Study the drawing (mm; zero at the part's minimum x, y, z) and answer. Round coordinates to 2 decimals unless told otherwise and drop trailing zeros. Write each loop counter-clockwise with the first axis right and the second up, starting at its lowest first coordinate (ties: lowest second). Pieces come first, ordered by that corner, then holes. Notation, with made-up numbers: (23, 60) - (75, 60) arc R25 cw to (75, 92) - close; hole circle Ø4 at (47.25, 55.25). An arc over 180 degrees is marked (long way). Return JSON: item names as keys, results as strings. Group by question number.
(1) Each of these flat-tipped pins is pushed along its axis until it touches: pin 1 (4 mm diameter, centred on x = 30, y = 20, fed in from +Z); pin 2 (8 mm diameter, centred on x = 30, y = 50, fed in from +Z). Where does it stop, or does it pass through?
(2) Section B-B, the plane z = 0.4 is taken. Give the number of separate pieces and of enclosed holes in the cut face, then the cut area to 3 significant figures.
(3) Section C-C, the plane y = 27.5 is taken. Write down the section's boundary in (x, z), then the cut area to 3 significant figures.
(4) Section A-A, the plane y = 59 is taken. Write down the section's boundary in (x, z), then the cut area to 3 significant figures.
(5) Find the intervals of material crossed by line 1 along X through (y, z) = (34.5, 1.45); line 2 along X through (y, z) = (51, 0.25), in increasing order. Write a range as [from, to].
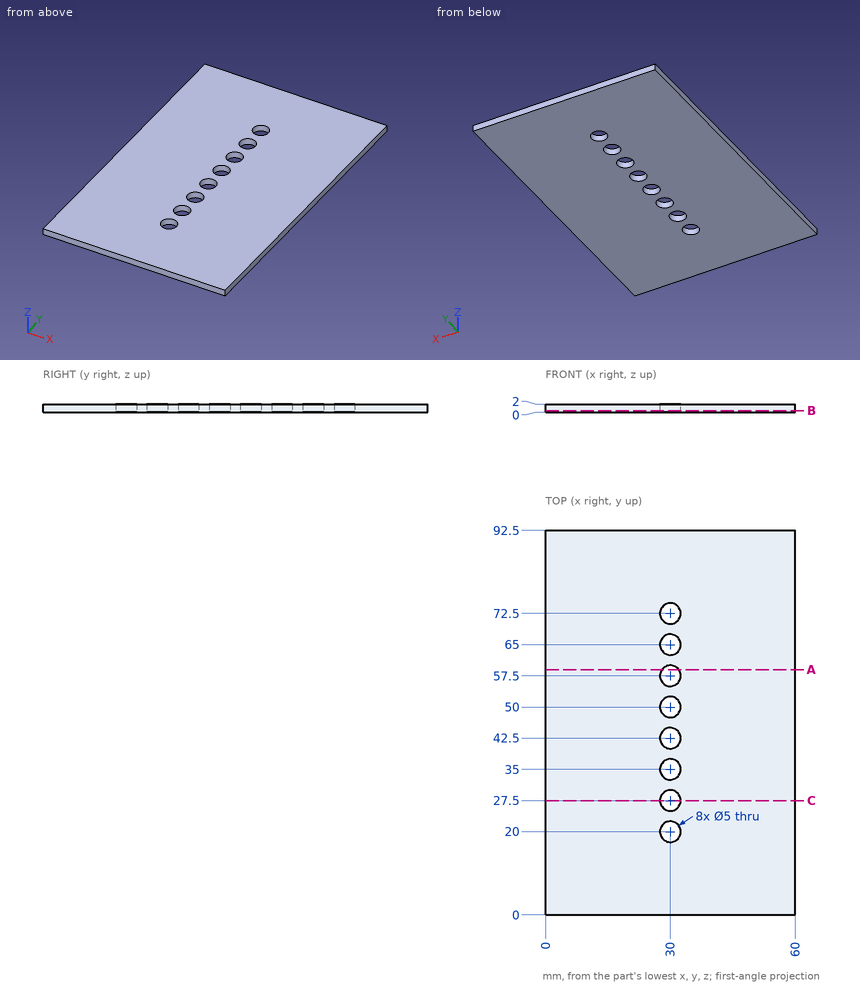
Working result:
{
 "1": {"pin 1": "passes through", "pin 2": "stops at z = 2"},
 "2": {"separate pieces": "1", "enclosed holes": "8", "area": "5,390 mm^2"},
 "3": {"outline": "(0, 0) - (27.5, 0) - (27.5, 2) - (0, 2) - close; (32.5, 0) - (60, 0) - (60, 2) - (32.5, 2) - close", "area": "110 mm^2"},
 "4": {"outline": "(0, 0) - (28, 0) - (28, 2) - (0, 2) - close; (32, 0) - (60, 0) - (60, 2) - (32, 2) - close", "area": "112 mm^2"},
 "5": {"line 1": "x = [0, 27.55], [32.45, 60]", "line 2": "x = [0, 27.71], [32.29, 60]"}
}
